Geometry: final body of the model. Coordinates: model frame, mm. A direction names the side the tool comes from. Round coordinates to 2 decimals unless told otherwise and drop trailing zeros. Loops run counter-clockwise (first coordinate to the right, second up) from the corner with the lowest first, then second, coordinate; pieces in that order, holes last. Notation, with made-up numbers: (65, 22) - (80, 22) arc R18 cw to (80, 49) - close; hole circle Ø9 at (33, 70). An arc over 180 degrees is marked (long way). Answer as a JSON object with one key per item and string values. Group by question number.
Item 1: Section C-C (y = 0). Return the cut outline in (x, z).
Item 2: Reachability of faces 4 (the face through (23.846, 7.509, 54.79)), 5 (the face through (-50, 0, 20)), 6 (the face through (-1, 27.5, 20)) from +Z, -Z, +X, -X, +Y, -Y: full face, straight path, thin tool, end or side. Return the list, or none.
Item 3: Section B-B (x = 40). Return the cut outline in (y, z).
Item 4: Draft query along Z for faces 1 (the face through (-1, -30, 20)), 2 (the face through (-1, 0, 2.5)), 3 (the face through (-22.34, 3.82, 70)). Return one class per face: released by +Z, released by -Z, zero draft, split by the parting line, or undercut.
Item 5: Section D-D (x = 5.5). Return the cut outline in (y, z).
Item 6: Line query: line 1 (Z direction, x = 17, y = 15); line 2 (X direction, y = 18, z = 31.5); line 3 (Y direction, x = -28, z = 25). Output: solid intervals per line, ascending.
Item 7: Section A-A (z = 13.5). Return the cut outline in (x, y).
Item 8: First-contact query: pin 1 (10 mm diameter, centred on x = -5.5, y = 12, fed in from +Z); pin 2 (12 mm diameter, centred on x = -14, z = 62.5, fed in from -Y); pin 3 (12 mm diameter, centred on x = -21.5, z = 47.5, fed in from +Y). Flat tips, straight axial feed; report the tip coordinate or a pass-through.
```python
from build123d import *

# Parameters (mm, degrees)
F0_W     = 100
F0_H     = 60
F1_DEPTH = 40
F2_R     = 25
F3_DEPTH = 30
F4_T     = -2.5


with BuildPart() as f1:
    # F0 (on Top) → F1 (new body)
    with BuildSketch(Plane.XY):
        Rectangle(F0_W, F0_H)
    extrude(amount=F1_DEPTH)

    # F2 (on face) → F3 (join)
    with BuildSketch(Plane.XY.offset(40)):
        Circle(F2_R)
    extrude(amount=F3_DEPTH)

    # F4
    f4_openings = [f1.faces().sort_by_distance(p)[0] for p in [
        (0, 0, 70),
    ]]
    offset(amount=F4_T, openings=f4_openings, kind=Kind.INTERSECTION)


solid = f1.part
```
Values:
{
 "1": {"outline": "(-50, 0) - (50, 0) - (50, 40) - (25, 40) - (25, 70) - (22.5, 70) - (22.5, 37.5) - (47.5, 37.5) - (47.5, 2.5) - (-47.5, 2.5) - (-47.5, 37.5) - (-22.5, 37.5) - (-22.5, 70) - (-25, 70) - (-25, 40) - (-50, 40) - close"},
 "2": {"face 4": "+Z", "face 5": "+Z, -Z, -X, +Y, -Y", "face 6": "none"},
 "3": {"outline": "(-30, 0) - (30, 0) - (30, 40) - (-30, 40) - close; hole (-27.5, 2.5) - (27.5, 2.5) - (27.5, 37.5) - (-27.5, 37.5) - close"},
 "4": {"face 1": "zero draft", "face 2": "undercut", "face 3": "released by +Z"},
 "5": {"outline": "(-30, 0) - (30, 0) - (30, 40) - (24.39, 40) - (24.39, 70) - (21.82, 70) - (21.82, 37.5) - (27.5, 37.5) - (27.5, 2.5) - (-27.5, 2.5) - (-27.5, 37.5) - (-21.82, 37.5) - (-21.82, 70) - (-24.39, 70) - (-24.39, 40) - (-30, 40) - close"},
 "6": {"line 1": "z = 0 to 2.5, 37.5 to 70", "line 2": "x = -50 to -47.5, 47.5 to 50", "line 3": "y = -30 to -27.5, 27.5 to 30"},
 "7": {"outline": "(-50, -30) - (50, -30) - (50, 30) - (-50, 30) - close; hole (-47.5, -27.5) - (47.5, -27.5) - (47.5, 27.5) - (-47.5, 27.5) - close"},
 "8": {"pin 1": "stops at z = 2.5", "pin 2": "stops at y = -23.69", "pin 3": "stops at y = 19.62"}
}
